```python
from build123d import *

# Parameters (mm, degrees)
BOSS_EXTRUDE1_DEPTH     = 50.8
SKETCH2_R               = 2.38125
CUT_EXTRUDE1_DEPTH      = 1
CUT_EXTRUDE1_DEPTH_BACK = 100.695
CUT_EXTRUDE2_DEPTH      = 96.340771022
CUT_EXTRUDE2_DEPTH_BACK = 94.451298519


with BuildPart() as part:
    # Sketch1 → Boss-Extrude1 (new body)
    with BuildSketch(Plane(origin=(0, 0, 0), x_dir=(1, 0, 0), z_dir=(0, 1, 0))):
        Polygon((-279.4, -117.475), (-182.668110184, 133.855439845), (-179.705, 132.715), (-275.9979581, -117.475), (-275.9979581, -132.715), (-279.4, -132.715), align=None)
    extrude(amount=BOSS_EXTRUDE1_DEPTH)

    # Sketch2 → Cut-Extrude1 (cut, two sides)
    with BuildSketch(Plane.ZY.offset(279.4)) as cut_extrude1_sk:
        with Locations((125.095, 25.4)):
            Circle(SKETCH2_R)
    extrude(amount=CUT_EXTRUDE1_DEPTH, mode=Mode.SUBTRACT)
    extrude(cut_extrude1_sk.sketch, amount=-CUT_EXTRUDE1_DEPTH_BACK, mode=Mode.SUBTRACT)

    # Sketch3 → Cut-Extrude2 (cut, two sides)
    with BuildSketch(Plane(origin=(-201.008455978, 0, -77.363998678), x_dir=(0.359193652, 0, -0.93326305), z_dir=(0.93326305, 0, 0.359193652))) as cut_extrude2_sk:
        with BuildLine():
            Line((-42.290889536, 50.8), (21.209110464, 50.8))
            ThreePointArc((21.209110464, 50.8), (-10.540889536, 43.18), (-42.290889536, 50.8))
        make_face()
        with BuildLine():
            Line((-42.290889536, 0), (21.209110464, 0))
            ThreePointArc((21.209110464, 0), (-10.540889536, 7.62), (-42.290889536, 0))
        make_face()
    extrude(amount=CUT_EXTRUDE2_DEPTH, mode=Mode.SUBTRACT)
    extrude(cut_extrude2_sk.sketch, amount=-CUT_EXTRUDE2_DEPTH_BACK, mode=Mode.SUBTRACT)


solid = part.part
```
CAD build for the part. Positions are in the model's coordinates, mm. A direction names the side the tool comes from. Coordinates: 2 decimals unless noted, no trailing zeros. Loops run counter-clockwise (first coordinate to the right, second up) from the corner with the lowest first, then second, coordinate; pieces in that order, holes last. Notation, with made-up numbers: (44.5, 13) - (56.5, 13) arc R16 ccw to (56.5, 42) - close; hole circle Ø8 at (-2.5, 22.5). An arc over 180 degrees is marked (long way). Return JSON: item names as keys, results as strings.
1. Band-saw the part on C-C (z = 53.5). Give the cut face in (x, y), and give its area (3 significant figures).
Result:
{"outline": "(-254.78, 0) - (-251.38, 0) - (-251.38, 50.8) - (-254.78, 50.8) - close", "area": "173 mm2"}
2. Band-saw the part on A-A (y = 25.4). Give the cut face in (x, z) (3 decimals).
Result:
{"outline": "(-279.4, 117.475) - (-182.668, -133.855) - (-179.705, -132.715) - (-275.998, 117.475) - (-275.998, 122.714) - (-279.4, 122.714) - close; (-279.4, 127.476) - (-275.998, 127.476) - (-275.998, 132.715) - (-279.4, 132.715) - close"}
3. 3-axis set-ups, long thin cutter, end or side, ignore diameter. For faces 1 (the flat face through (-275.998, 25, 122)), 2 (the flat face through (-250, 50.8, 46)): which of +Z, -Z, +X, -X, +Y, -Y reach the whole face in a straight line?
Result:
{"face 1": "+Z, +X, +Y, -Y", "face 2": "+Z, -Z, +X, -X, +Y"}
4. Probe L1, parallel to X at y = 44.5, z = -114; L2, parallel to X at y = 27.5, z = 36.5. List the from-to ranges inside material, lowest first. Write a range as from..to.
Result:
{"L1": "x = -190.31..-186.91", "L2": "x = -248.23..-244.83"}
5. Band-saw the part on D-D (x = -251). Give the cut face in (y, z), and give its area (3 significant figures).
Result:
{"outline": "(0, 43.69) - (50.8, 43.69) - (50.8, 52.52) - (0, 52.52) - close", "area": "449 mm2"}
6. Band-saw the part on B-B (y = 11). Give the cut face in (x, z) (3 decimals).
Result:
{"outline": "(-279.4, 117.475) - (-182.668, -133.855) - (-179.705, -132.715) - (-275.998, 117.475) - (-275.998, 132.715) - (-279.4, 132.715) - close"}
7. Drop flat-ended pins along their axis: pin 1 (8 mm diameter, centred on y = 32, z = 34.5, fed in from -X); pin 2 (1.5 mm diameter, centred on y = 19, z = 27, fed in from +X); pin 3 (7.5 mm diameter, centred on y = 33.5, z = 127, fed in from +X). Give the stop position or say it passes through.
Result:
{"pin 1": "stops at x = -249", "pin 2": "stops at x = -240.89", "pin 3": "stops at x = -276"}
